```python
from build123d import *

# Parameters (mm, degrees)
SKETCH1_W                       = 25.4
SKETCH1_H                       = 50.8
SKETCH1_W_2                     = 19.05
SKETCH1_H_2                     = 44.45
EXTRUDE_THIN1_DEPTH             = 501.65
F_3_16_0_1875_DIAMETER_HOLE1_D  = 4.7625
F_1_4_0_25_DIAMETER_HOLE1_D     = 6.35
F_1_4_0_25_DIAMETER_HOLE1_DEPTH = 25.4
F_1_4_0_25_DIAMETER_HOLE1_TIP   = 1.907732465
F_1_4_CLEARANCE_HOLE1_D         = 6.7564
F_1_4_CLEARANCE_HOLE1_DEPTH     = 38.1
F_1_4_CLEARANCE_HOLE1_TIP       = 2.029827343
F_3_16_0_195_DIAMETER_HOLE1_D   = 4.953


with BuildPart() as part:
    # Sketch1 → Extrude-Thin1 (new body)
    with BuildSketch(Plane.XY):
        Rectangle(SKETCH1_W, SKETCH1_H)
        Rectangle(SKETCH1_W_2, SKETCH1_H_2, mode=Mode.SUBTRACT)
    extrude(amount=EXTRUDE_THIN1_DEPTH)

    # 3/16 (0.1875) Diameter Hole1 (through all)
    with Locations(Plane(origin=(0, 25.4, 495.3), x_dir=(1, 0, 0), z_dir=(0, 1, 0))):
        with Locations((0, 0), (0, 488.95), (0, 463.55), (0, 438.15), (0, 25.4), (0, 50.8)):
            Hole(F_3_16_0_1875_DIAMETER_HOLE1_D / 2)

    # 1/4 (0.25) Diameter Hole1
    with Locations(Plane(origin=(0, 25.4, 0), x_dir=(1, 0, 0), z_dir=(0, 1, 0))):
        with Locations((0, -79.831), (0, -425.933853021), (0, -327.499040355), (0, -200.481)):
            Hole(F_1_4_0_25_DIAMETER_HOLE1_D / 2, depth=F_1_4_0_25_DIAMETER_HOLE1_DEPTH)
            with Locations((0, 0, -(F_1_4_0_25_DIAMETER_HOLE1_DEPTH + F_1_4_0_25_DIAMETER_HOLE1_TIP / 2))):  # 118° drill point
                Cone(0, F_1_4_0_25_DIAMETER_HOLE1_D / 2, F_1_4_0_25_DIAMETER_HOLE1_TIP, mode=Mode.SUBTRACT)

    # 1/4 Clearance Hole1
    with Locations(Plane(origin=(381, 25.4, 250.825), x_dir=(1, 0, 0), z_dir=(0, 1, 0))):
        with Locations((381, 82.55), (381, 98.425), (381, 114.3), (381, -146.05), (381, -130.175), (381, -114.3), (-381, -146.05), (-381, -130.175), (-381, -114.3), (-381, 82.55), (-381, 98.425), (-381, 114.3)):
            Hole(F_1_4_CLEARANCE_HOLE1_D / 2, depth=F_1_4_CLEARANCE_HOLE1_DEPTH)
            with Locations((0, 0, -(F_1_4_CLEARANCE_HOLE1_DEPTH + F_1_4_CLEARANCE_HOLE1_TIP / 2))):  # 118° drill point
                Cone(0, F_1_4_CLEARANCE_HOLE1_D / 2, F_1_4_CLEARANCE_HOLE1_TIP, mode=Mode.SUBTRACT)

    # 3/16 (0.195) Diameter Hole1 (through all)
    with Locations(Plane(origin=(0, -25.4, 0), x_dir=(-1, 0, 0), z_dir=(0, -1, 0))):
        with Locations((3.169336228, -85.725), (-3.180663772, -111.125), (3.169336228, -136.525), (-3.180663772, -161.925), (3.169336228, -187.325), (-3.180663772, -212.725), (3.169336228, -238.125), (-3.180663772, -263.525), (3.169336228, -288.925), (-3.180663772, -314.325), (3.169336228, -339.725), (-3.180663772, -365.125), (3.169336228, -390.525), (-3.180663772, -415.925)):
            Hole(F_3_16_0_195_DIAMETER_HOLE1_D / 2)


solid = part.part
```
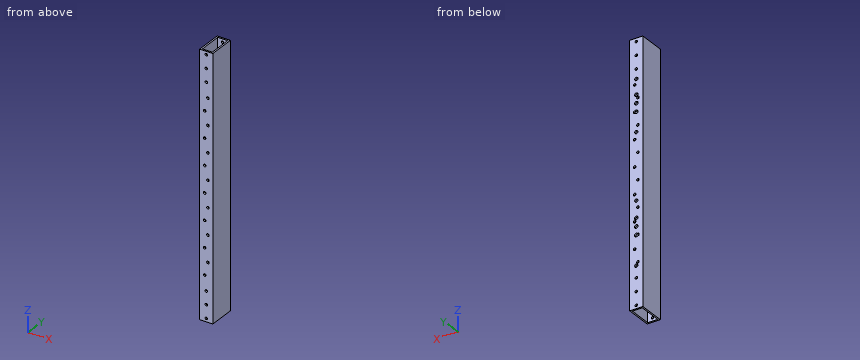
Part model, mm, in its own coordinate system. Round coordinates to 2 decimals unless told otherwise and drop trailing zeros. Loops run counter-clockwise (first coordinate to the right, second up) from the corner with the lowest first, then second, coordinate; pieces in that order, holes last.
Item 1: Cut at B-B, the plane y = 11. Give the cut face in (x, z) (3 decimals), then the cut area to 3 significant figures.
Item 2: Drill centre lines: line 1 (Y direction, x = -1.25, z = 376.5) (3 decimals); line 2 (X direction, y = -5.5, z = 387) (3 decimals); line 3 (X direction, y = 23, z = 152.4). Where is each one in solid material? Low to high.
Item 3: Drop a flat-ended pin along its axis: P1, Ø4.5, axis at x = 3.18, z = 111.12, coming from the -Y side. Give the stop position or say it passes through.
Item 4: Cut at A-A, the plane z = 434.5. Give the cut face in (x, y) (3 decimals).
A:
1. outline: (-12.7, 0) - (-9.525, 0) - (-9.525, 501.65) - (-12.7, 501.65) - close; (9.525, 0) - (12.7, 0) - (12.7, 501.65) - (9.525, 501.65) - close
1. area: 3,190 mm2
2. line 1: y = -25.4 to -22.225, 22.225 to 25.4
2. line 2: x = -12.7 to -9.525, 9.525 to 12.7
2. line 3: x = -12.7 to -3.38, 3.38 to 12.7
3. P1: passes through
4. outline: (-12.7, -25.4) - (12.7, -25.4) - (12.7, 25.4) - (-12.7, 25.4) - close; hole (-9.525, -22.225) - (9.525, -22.225) - (9.525, 22.225) - (-9.525, 22.225) - close
